Part model, mm, in its own coordinate system. A direction names the side the tool comes from. Round coordinates to 2 decimals unless told otherwise and drop trailing zeros. Write each loop counter-clockwise with the first axis right and the second up, starting at its lowest first coordinate (ties: lowest second). Pieces come first, ordered by that corner, then holes.
```python
from build123d import *

# Parameters (mm, degrees)
F1_DEPTH    = 20
F3_DEPTH    = 5
F4_W        = 10
F4_H        = 10
F5_DEPTH    = 5
F6_D        = 5
F7_D        = 5
F8_T1_DEPTH = 25


# Not quite as in the source:
# - a fillet or chamfer that OpenCascade refuses, or shapes differently, is made with other operations: its cross-section is extruded or revolved along the edge and cut away or added


with BuildPart() as f1:
    # F0 (on Top) → F1 (new body)
    with BuildSketch(Plane.XY):
        with BuildLine():
            Line((16.7705098646, 4.9999998882), (53.0298836529, 4.9999998882))
            Line((53.0298836529, 4.9999998882), (53.0298836529, 34.6554927528))
            Line((53.0298836529, 34.6554927528), (5, 34.6554927528))
            Line((5, 34.6554927528), (5, 16.7705098312))
            ThreePointArc((5, 16.7705098312), (12.374368712, 12.3743686295), (16.7705098646, 4.9999998882))
        make_face()
        with BuildLine():
            Line((5, 16.7705098312), (5, 34.6554927528))
            Line((5, 34.6554927528), (-5, 34.6554927528))
            Line((-5, 34.6554927528), (-5, 16.7705098312))
            ThreePointArc((-5, 16.7705098312), (0, 17.5), (5, 16.7705098312))
        make_face()
        with BuildLine():
            Line((-53.0298836529, 34.6554927528), (-53.0298836529, 4.9999998882))
            Line((-53.0298836529, 4.9999998882), (-16.7705098646, 4.9999998882))
            ThreePointArc((-16.7705098646, 4.9999998882), (-12.374368712, 12.3743686295), (-5, 16.7705098312))
            Line((-5, 16.7705098312), (-5, 34.6554927528))
            Line((-5, 34.6554927528), (-53.0298836529, 34.6554927528))
        make_face()
        with BuildLine():
            Line((-53.0298836529, -34.6554927528), (-5, -34.6554927528))
            Line((-5, -34.6554927528), (-5, -16.7705098312))
            ThreePointArc((-5, -16.7705098312), (-12.374368712, -12.3743686295), (-16.7705098646, -4.9999998882))
            Line((-16.7705098646, -4.9999998882), (-53.0298836529, -4.9999998882))
            Line((-53.0298836529, -4.9999998882), (-53.0298836529, -34.6554927528))
        make_face()
        with BuildLine():
            Line((5, -34.6554927528), (53.0298836529, -34.6554927528))
            Line((53.0298836529, -34.6554927528), (53.0298836529, -4.9999998882))
            Line((53.0298836529, -4.9999998882), (16.7705098646, -4.9999998882))
            ThreePointArc((16.7705098646, -4.9999998882), (12.374368712, -12.3743686295), (5, -16.7705098312))
            Line((5, -16.7705098312), (5, -34.6554927528))
        make_face()
        with BuildLine():
            Line((16.7705098646, -4.9999998882), (53.0298836529, -4.9999998882))
            Line((53.0298836529, -4.9999998882), (53.0298836529, 4.9999998882))
            Line((53.0298836529, 4.9999998882), (16.7705098646, 4.9999998882))
            ThreePointArc((16.7705098646, 4.9999998882), (17.3166671538, 2.5264676299), (17.5, 0))
            ThreePointArc((17.5, 0), (17.3166671538, -2.5264676299), (16.7705098646, -4.9999998882))
        make_face()
        with BuildLine():
            ThreePointArc((-5, -16.7705098312), (0, -17.5), (5, -16.7705098312))
            ThreePointArc((5, -16.7705098312), (12.374368712, -12.3743686295), (16.7705098646, -4.9999998882))
            ThreePointArc((16.7705098646, -4.9999998882), (17.3166671538, -2.5264676299), (17.5, 0))
            ThreePointArc((17.5, 0), (17.3166671538, 2.5264676299), (16.7705098646, 4.9999998882))
            ThreePointArc((16.7705098646, 4.9999998882), (12.374368712, 12.3743686295), (5, 16.7705098312))
            ThreePointArc((5, 16.7705098312), (0, 17.5), (-5, 16.7705098312))
            ThreePointArc((-5, 16.7705098312), (-12.374368712, 12.3743686295), (-16.7705098646, 4.9999998882))
            ThreePointArc((-16.7705098646, 4.9999998882), (-17.5, 0), (-16.7705098646, -4.9999998882))
            ThreePointArc((-16.7705098646, -4.9999998882), (-12.374368712, -12.3743686295), (-5, -16.7705098312))
        make_face()
        with BuildLine():
            Line((-53.0298836529, 4.9999998882), (-53.0298836529, -4.9999998882))
            Line((-53.0298836529, -4.9999998882), (-16.7705098646, -4.9999998882))
            ThreePointArc((-16.7705098646, -4.9999998882), (-17.5, 0), (-16.7705098646, 4.9999998882))
            Line((-16.7705098646, 4.9999998882), (-53.0298836529, 4.9999998882))
        make_face()
        with BuildLine():
            Line((-5, -34.6554927528), (5, -34.6554927528))
            Line((5, -34.6554927528), (5, -16.7705098312))
            ThreePointArc((5, -16.7705098312), (0, -17.5), (-5, -16.7705098312))
            Line((-5, -16.7705098312), (-5, -34.6554927528))
        make_face()
    extrude(amount=F1_DEPTH)

    # F2 (on face) → F3 (cut)
    with BuildSketch(Plane.XY.offset(20)):
        with BuildLine():
            Line((-52.9048836529, 4.9999998882), (-52.9048836529, -4.9999998882))
            Line((-52.9048836529, -4.9999998882), (-16.6455098646, -4.9999998882))
            ThreePointArc((-16.6455098646, -4.9999998882), (-17.375, 0), (-16.6455098646, 4.9999998882))
            Line((-16.6455098646, 4.9999998882), (-52.9048836529, 4.9999998882))
        make_face()
        with BuildLine():
            ThreePointArc((-4.875, 16.7705098312), (0.125, 17.5), (5.125, 16.7705098312))
            Line((5.125, 16.7705098312), (5.125, 34.6554927528))
            Line((5.125, 34.6554927528), (-4.875, 34.6554927528))
            Line((-4.875, 34.6554927528), (-4.875, 16.7705098312))
        make_face()
        with BuildLine():
            ThreePointArc((-4.875, -16.7705098312), (0.125, -17.5), (5.125, -16.7705098312))
            ThreePointArc((5.125, -16.7705098312), (12.499368712, -12.3743686295), (16.8955098646, -4.9999998882))
            ThreePointArc((16.8955098646, -4.9999998882), (17.4416671538, -2.5264676299), (17.625, 0))
            ThreePointArc((17.625, 0), (17.4416671538, 2.5264676299), (16.8955098646, 4.9999998882))
            ThreePointArc((16.8955098646, 4.9999998882), (12.499368712, 12.3743686295), (5.125, 16.7705098312))
            ThreePointArc((5.125, 16.7705098312), (0.125, 17.5), (-4.875, 16.7705098312))
            ThreePointArc((-4.875, 16.7705098312), (-12.249368712, 12.3743686295), (-16.6455098646, 4.9999998882))
            ThreePointArc((-16.6455098646, 4.9999998882), (-17.375, 0), (-16.6455098646, -4.9999998882))
            ThreePointArc((-16.6455098646, -4.9999998882), (-12.249368712, -12.3743686295), (-4.875, -16.7705098312))
        make_face()
        with BuildLine():
            Line((16.8955098646, -4.9999998882), (53.0298836529, -4.9999998882))
            Line((53.0298836529, -4.9999998882), (53.0298836529, 4.9999998882))
            Line((53.0298836529, 4.9999998882), (16.8955098646, 4.9999998882))
            ThreePointArc((16.8955098646, 4.9999998882), (17.4416671538, 2.5264676299), (17.625, 0))
            ThreePointArc((17.625, 0), (17.4416671538, -2.5264676299), (16.8955098646, -4.9999998882))
        make_face()
        with BuildLine():
            Line((-4.875, -34.6554927528), (5.125, -34.6554927528))
            Line((5.125, -34.6554927528), (5.125, -16.7705098312))
            ThreePointArc((5.125, -16.7705098312), (0.125, -17.5), (-4.875, -16.7705098312))
            Line((-4.875, -16.7705098312), (-4.875, -34.6554927528))
        make_face()
    extrude(amount=-F3_DEPTH, mode=Mode.SUBTRACT)

    # F4 (on face) → F5 (cut)
    with BuildSketch(Plane.XY.offset(20)):
        with Locations((-29.0774418265, 25.713001292)):
            Rectangle(F4_W, F4_H)
        with Locations((29.0774418265, 25.713001292)):
            Rectangle(F4_W, F4_H)
        with Locations((29.0774418265, -25.713001292)):
            Rectangle(F4_W, F4_H)
        with Locations((-29.0774418265, -25.713001292)):
            Rectangle(F4_W, F4_H)
    extrude(amount=-F5_DEPTH, mode=Mode.SUBTRACT)

    # F6 (through all)
    with Locations(Plane(origin=(0, 0, 0), x_dir=(1, 0, 0), z_dir=(0, 0, -1))):
        with Locations((0, 34.6554927528), (0, -34.6554927528), (-53.0298836529, 0), (0, 0)):
            Hole(F6_D / 2)

    # F7 (through all)
    with Locations(Plane(origin=(0, 0, 0), x_dir=(1, 0, 0), z_dir=(0, 0, -1))):
        with Locations((53.0298836529, 0)):
            Hole(F7_D / 2)

    # F8: fillet of radius 1 on 4 edges, made by hand

    # F8_s2 → F8_t1 (cut)
    with BuildSketch(Plane.XY.offset(-2.5)):
        with BuildLine():
            add(Edge.make_bspline(
                [(52.0298836529, -34.6554927528), (53.0298836529, -34.6554927528), (53.0298836529, -33.6554927528)],
                knots=[0, 0, 0, 1, 1, 1], degree=2, weights=[1, 1, 1]))
            Line((53.0298836529, -33.6554927528), (53.0298836529, -34.6554927528))
            Line((53.0298836529, -34.6554927528), (52.0298836529, -34.6554927528))
        make_face()
        with BuildLine():
            add(Edge.make_bspline(
                [(52.0298836529, 34.6554927528), (53.0298836529, 34.6554927528), (53.0298836529, 33.6554927528)],
                knots=[0, 0, 0, 1, 1, 1], degree=2, weights=[1, 1, 1]))
            Line((53.0298836529, 33.6554927528), (53.0298836529, 34.6554927528))
            Line((53.0298836529, 34.6554927528), (52.0298836529, 34.6554927528))
        make_face()
        with BuildLine():
            add(Edge.make_bspline(
                [(-52.0298836529, -34.6554927528), (-53.0298836529, -34.6554927528), (-53.0298836529, -33.6554927528)],
                knots=[0, 0, 0, 1, 1, 1], degree=2, weights=[1, 1, 1]))
            Line((-53.0298836529, -33.6554927528), (-53.0298836529, -34.6554927528))
            Line((-53.0298836529, -34.6554927528), (-52.0298836529, -34.6554927528))
        make_face()
        with BuildLine():
            add(Edge.make_bspline(
                [(-53.0298836529, 33.6554927528), (-53.0298836529, 34.6554927528), (-52.0298836529, 34.6554927528)],
                knots=[0, 0, 0, 1, 1, 1], degree=2, weights=[1, 1, 1]))
            Line((-52.0298836529, 34.6554927528), (-53.0298836529, 34.6554927528))
            Line((-53.0298836529, 34.6554927528), (-53.0298836529, 33.6554927528))
        make_face()
    extrude(amount=F8_T1_DEPTH, mode=Mode.SUBTRACT)


solid = f1.part
```
Q1. Which spindle directions (+Z, -Z, +X, -X, +Y, -Y) get a long thin tool onto all of the face, cutting with end or side? Do faces 5 (the flat face through (-4.875, -26, 18)), 6 (the flat face through (-29, -20.713, 18)), 7 (the flat face through (35, -5, 18)). Say none if no direction does.
Values follow:
face 5: +Z, +Y, -Y
face 6: +Z
face 7: +Z, +X
Q2. Cut at A-A on x = 0. Write the cut outline in (y, z).
Values follow:
outline: (-32.16, 0) - (-2.5, 0) - (-2.5, 15) - (-32.16, 15) - close; (2.5, 0) - (32.16, 0) - (32.16, 15) - (2.5, 15) - close
Q3. Mould opens along Y. For faces 1 (the flat face through (24.077, 26, 18)), 2 (the flat face through (-29, -26, 15)), 3 (the flat face through (5.125, 26, 18)), 4 (the cylindrical face through (0.055, -32.156, 7.605)) say: +Y half, -Y half, draft (parallel to the pull), parting line (faces both ways), or undercut.
Values follow:
face 1: undercut
face 2: undercut
face 3: draft
face 4: -Y half
Q4. Drop a flat-ended pin along its axis: pin 1 (3 mm diameter, centred on x = -29.5, y = 27.5, fed in from +Z). Give the stop position or say it passes through.
Values follow:
pin 1: stops at z = 15
Q5. Cut at D-D on x = -37. Write the cut outline in (y, z), plus the area to 3 significant figures.
Values follow:
outline: (-34.66, 0) - (34.66, 0) - (34.66, 20) - (5, 20) - (5, 15) - (-5, 15) - (-5, 20) - (-34.66, 20) - close
area: 1,340 mm2
Q6. Wall check: L1, parallel to X at y = 27, z = 19.25 (3 decimals); L2, parallel to Y at x = 0, z = 10; L3, parallel to Y at x = 45, z = 16. Give the ranges that are in metal, low to high.
Values follow:
L1: x = -53.03 to -34.077, -24.077 to -4.875, 5.125 to 24.077, 34.077 to 53.03
L2: y = -32.16 to -2.5, 2.5 to 32.16
L3: y = -34.66 to -5, 5 to 34.66
Q7. Cut at C-C on y = 0. Write the cut outline in (x, z), plus the area to 3 significant figures.
Values follow:
outline: (-50.53, 0) - (-2.5, 0) - (-2.5, 15) - (-50.53, 15) - close; (2.5, 0) - (50.53, 0) - (50.53, 15) - (2.5, 15) - close
area: 1,440 mm2
Q8. Cut at B-B on z = 18.25. State how many separate pieces and enclosed holes the cut face has, plus the area to 3 significant figures.
Values follow:
separate pieces: 4
enclosed holes: 4
area: 4,930 mm2
